Part model, mm, in its own coordinate system. Face numbers are marked on the shaded views. Round coordinates to 2 decimals unless told otherwise and drop trailing zeros. Order: outer loops, then holes, each group sorted by start corner. A loop starts at its lowest first (then second) coordinate and runs counter-clockwise, first axis right, second up. Notation, with made-up numbers: M 44.25,12.25 L 48.25,12.25 A13 cw 48.25,16.25 Z; hole C 61,-27 d1. An arc over 180 degrees is marked long. Write each question's results on one line, items separated by ' | '. Start each with the question number.
1. Drop flat-ended pins along their axis: pin 1 Ø5 at (x, z) = (-39, 11) entering from -Y; pin 2 Ø1.2 at (x, z) = (3, 18) entering from +Y; pin 3 Ø2 at (y, z) = (57.5, 17) entering from -X. Give the stop position or say it passes through.
2. Two-plate mould, pull along X, no slides. Class the marked faces 1, 2, 3 and 4: +X half, -X half, draft (parallel to the pull), parting line (faces both ways), or undercut.
3. Band-saw the part on A-A, the plane y = 38. List the corners of the cut face in (x, z).
4. Band-saw the part on B-B, the plane x = -19.5. List the corners of the cut face in (y, z).
5. Probe L1, parallel to Z at x = -104, y = 5; L2, parallel to X at y = 8, z = 6.5; L3, parallel to Y at x = -103.45, z = 19. List the from-to ranges inside material, lowest first. Write a range as [from, to].
6. Band-saw the part on C-C, the plane y = 14. List the corners of the cut face in (x, z).
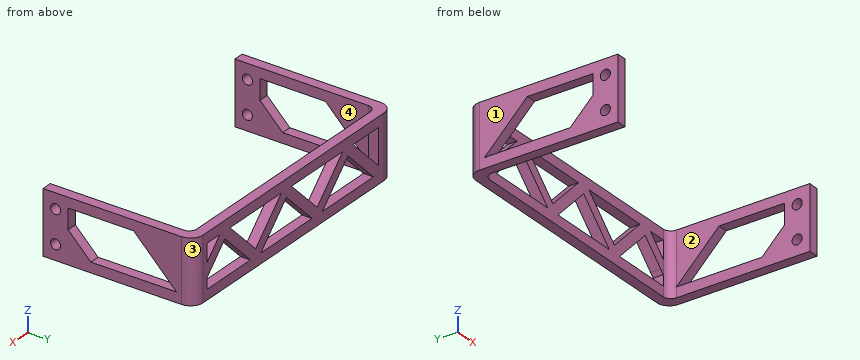
```python
from build123d import *

# Parameters (mm, degrees)
F1_DEPTH = 25
F3_DEPTH = 25
F5_DEPTH = 200


with BuildPart() as f1:
    # F0 (on Top) → F1 (new body)
    with BuildSketch(Plane.XY):
        with BuildLine():
            Line((0, 53), (0, 0))
            Line((0, 0), (4, 0))
            Line((4, 0), (4, 55))
            ThreePointArc((4, 55), (2.5355339059, 58.5355339059), (-1, 60))
            Line((-1, 60), (-101, 60))
            ThreePointArc((-101, 60), (-104.5355339059, 58.5355339059), (-106, 55))
            Line((-106, 55), (-106, 0))
            Line((-106, 0), (-102, 0))
            Line((-102, 0), (-102, 53))
            ThreePointArc((-102, 53), (-101.1213203436, 55.1213203436), (-99, 56))
            Line((-99, 56), (-3, 56))
            ThreePointArc((-3, 56), (-0.8786796564, 55.1213203436), (0, 53))
        make_face()
    extrude(amount=F1_DEPTH)

    # F2 (on face) → F3 (cut)
    with BuildSketch(Plane.XZ.offset(-56)):
        Polygon((-49.8284271247, 21), (-78.1715728753, 21), (-64, 6.8284271247), align=None)
        Polygon((-30, 6.8284271247), (-15.8284271247, 21), (-44.1715728753, 21), align=None)
        Polygon((-95.1715728753, 4), (-66.8284271247, 4), (-81, 18.1715728753), align=None)
        Polygon((-10.1715728753, 21), (-3, 13.8284271247), (-3, 21), align=None)
        Polygon((-98, 21), (-98, 6.8284271247), (-83.8284271247, 21), align=None)
        Polygon((-61.1715728753, 4), (-32.8284271247, 4), (-47, 18.1715728753), align=None)
        Polygon((-4.4142135624, 9.5857864376), (-13, 18.1715728753), (-27.1715728753, 4), (-3, 4), (-3, 8.1715728753), align=None)
    extrude(amount=-F3_DEPTH, mode=Mode.SUBTRACT)

    # F4 (on face) → F5 (cut)
    with BuildSketch(Plane(origin=(-106, 0, 0), x_dir=(0, -1, 0), z_dir=(-1, 0, 0))):
        with BuildLine():
            ThreePointArc((-5, 21), (-6.4142135624, 17.5857864376), (-3, 19))
            ThreePointArc((-3, 19), (-3.5857864376, 20.4142135624), (-5, 21))
        make_face()
        with BuildLine():
            ThreePointArc((-3, 6), (-6.4142135624, 7.4142135624), (-5, 4))
            ThreePointArc((-5, 4), (-3.5857864376, 4.5857864376), (-3, 6))
        make_face()
        Polygon((-10, 13), (-10, 21), (-36, 21), (-19, 4), align=None)
        Polygon((-19, 4), (-36, 21), (-53, 4), align=None)
    extrude(amount=-F5_DEPTH, mode=Mode.SUBTRACT)


solid = f1.part
```
Solution:
1) pin 1: y = 56 | pin 2: y = 58.67 | pin 3: x = -105.77
2) face 1: -X half | face 2: undercut | face 3: +X half | face 4: undercut
3) outline: M -106,0 L -102,0 L -102,4 L -106,4 Z; M -106,19 L -102,19 L -102,25 L -106,25 Z; M 0,0 L 4,0 L 4,4 L 0,4 Z; M 0,19 L 4,19 L 4,25 L 0,25 Z
4) outline: M 56,0 L 60,0 L 60,4 L 56,4 Z; M 56,11.67 L 60,11.67 L 60,17.33 L 56,17.33 Z; M 56,21 L 60,21 L 60,25 L 56,25 Z
5) L1: [0, 4], [8, 17], [21, 25] | L2: [-106, -102], [0, 4] | L3: [0, 3], [7, 10], [38, 59.36]
6) outline: M -106,0 L -102,0 L -102,9 L -106,9 Z; M -106,21 L -102,21 L -102,25 L -106,25 Z; M 0,0 L 4,0 L 4,9 L 0,9 Z; M 0,21 L 4,21 L 4,25 L 0,25 Z
